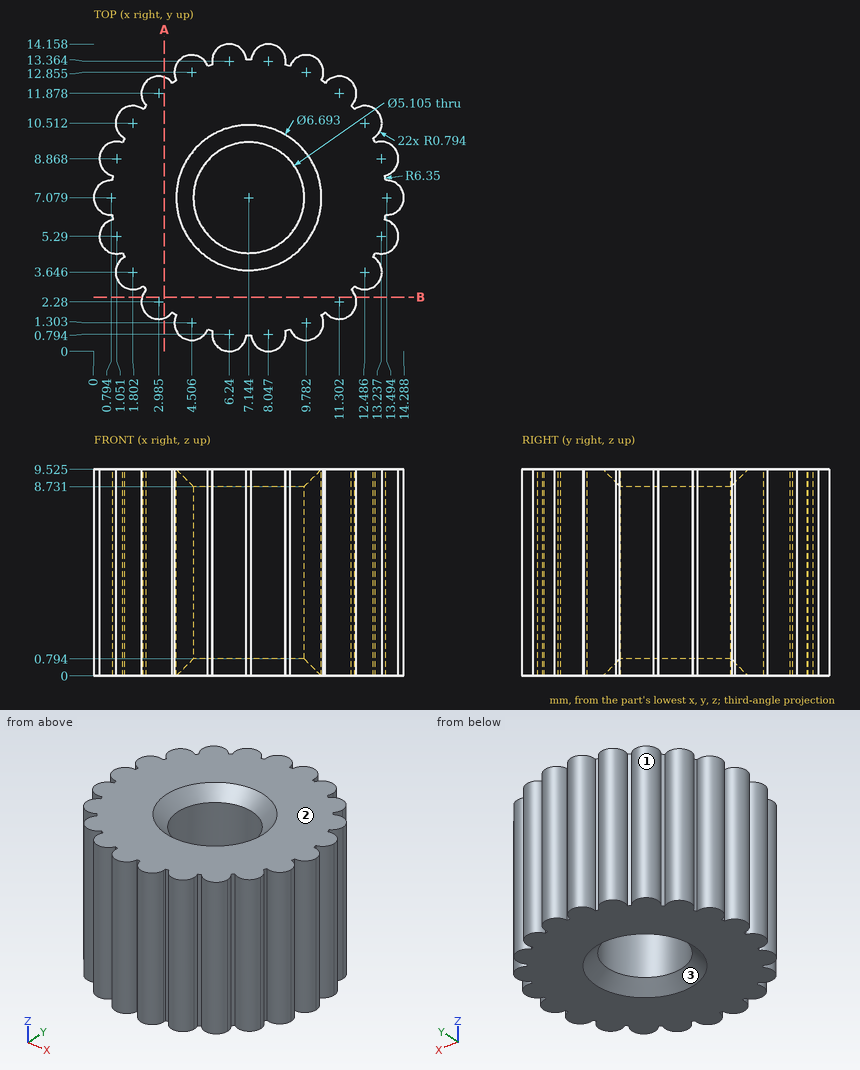
Print and shaded views of the part. All mm, measured from the part's lowest x, y and z. Coordinates: 2 decimals unless noted, no trailing zeros. Loops run counter-clockwise (first coordinate to the right, second up) from the corner with the lowest first, then second, coordinate; pieces in that order, holes last. Notation, with made-up numbers: (0.25, -13.75) -> (41.25, -13.75) arc R26 cw to (41.25, 6.25) -> close; hole circle Ø10 at (89, 78). An arc over 180 degrees is marked (long way). Use a Markdown table: item, result. Add a question column.
Item 1: Band-saw the part on B-B on y = 2.5. Write the cut outline in (x, z) (1 decimal).
Item 2: Flat gauge pins, fed straight in: P1, Ø6, axis at x = 4, y = 6.5, coming from the +Z side (1 decimal); P2, Ø4, axis at y = 10.5, z = 5, coming from the +X side. Where does each tip first touch, or does it go through?
Item 3: Probe probe 1 along Y at (x, z) = (1.25, 5.25) (1 decimal); probe 2 along Y at (x, z) = (3, 3.5); probe 3 along X at (y, z) = (2.25, 3.5) (1 decimal). List the from-to ranges inside material, lowest first.
Item 4: Band-saw the part on A-A on x = 3.25. Write the cut outline in (y, z) (1 decimal).
Item 5: Pull direction X, two halves, no side cores. Call the marked faces 1, 2 and 3: +X half, -X half, draft (parallel to the pull), parting line (faces both ways), or undercut.
Geometry says:
| question | item | result |
|---|---|---|
| 1 | outline | (2.2, 0) -> (12.1, 0) -> (12.1, 9.5) -> (2.2, 9.5) -> close |
| 2 | P1 | z = 9.5 |
| 2 | P2 | x = 14.03 |
| 3 | probe 1 | 3.1 to 4.2, 4.5 to 9.6, 9.9 to 11.1 |
| 3 | probe 2 | 1.49 to 12.67 |
| 3 | probe 3 | 2.2 to 12.1 |
| 4 | outline | (1.5, 0) -> (12.6, 0) -> (12.6, 9.5) -> (1.5, 9.5) -> close |
| 5 | face 1 | undercut |
| 5 | face 2 | draft |
| 5 | face 3 | undercut |
